Autodesk Inventor part; units mm, degrees
ref_plane "Work Plane1" through (-12.5, 0, 453) normal (1, 0, 0) x (0, 1, 0)
ref_plane "XZ Plane" through (0, 0, 0) normal (0, 1, 0) x (-1, 0, 0)
ref_plane "XY Plane" through (0, 0, 0) normal (0, 0, 1) x (1, 0, 0)
sketch "Sketch2" plane through (0, 0, 0) normal (0, 1, 0) x (-1, 0, 0)
  line L0 (0, 0) -> (0, 513)
  line L1 (0, 513) -> (-12.5, 513)
  line L2 (-12.5, 513) -> (-12.5, 393)
  line L3 (-19, 393) -> (-19, 308)
  line L4 (-19, 308) -> (-15, 308)
  line L5 (-15, 308) -> (-15, 0)
  line L6 (-15, 0) -> (0, 0)
  line L7 (-19, 393) -> (-12.5, 393)
  dimension "d6" = 30
  dimension "d11" = 308
  dimension "d12" = 85
  dimension "d13" = 120
  dimension "d14" = 38
  dimension "d15" = 25
revolve "Revolution1" add sketch "Sketch2" angle 360 about axis through (0, 0, 0) along (0, 0, 1)
ref_plane "Work Plane1" through (-12.5, 0, 453) normal (1, 0, 0) x (0, 1, 0)
sketch "Sketch3" plane through (-12.5, 0, 453) normal (1, 0, 0) x (0, 1, 0)
  line L0 (12.5, -60) -> (-12.5, -60)
  line L1 (12.5, 60) -> (-12.5, 60)
  line L2 (0.1403, 48) -> (0.1403, 38) construction
  line L3 (-3.8597, 48) -> (-3.8597, 38)
  line L4 (4.1403, 38) -> (4.1403, 48)
  arc A0 (4.1403, 48) -> (-3.8597, 48) centre (0.1403, 48) ccw
  arc A1 (-3.8597, 38) -> (4.1403, 38) centre (0.1403, 38) ccw
  point P0 (0, -453)
  point P1 (0.1403, 43)
  dimension "d8" = 12
  dimension "d9" = 8
  dimension "d10" = 10
extrude "Extrusion2" cut sketch "Sketch3" along normal blind 10
properties part number "NVPH-312 augur shaft"
CAD build for the part. Positions are in the model's coordinates, mm. A direction names the side the tool comes from. Round coordinates to 2 decimals unless told otherwise and drop trailing zeros. Write each loop counter-clockwise with the first axis right and the second up, starting at its lowest first coordinate (ties: lowest second). Pieces come first, ordered by that corner, then holes.
Item 1: Mould opens along Z. For faces 1 (the cylindrical face through (8.767, 16.856, 349.905)), 2 (the flat face through (0, 0, 0)), 3 (the flat face through (0, 0, 513)), 4 (the flat face through (-2.5, 0, 496)) say: released by +Z, released by -Z, zero draft, split by the parting line, or undercut.
Filled in:
face 1: zero draft
face 2: released by -Z
face 3: released by +Z
face 4: undercut
Item 2: Band-saw the part on B-B on z = 416.5. Write the cut outline in (x, y), then the cut area to 3 significant figures.
Filled in:
outline: circle Ø25 at (0, 0)
area: 491 mm2
Item 3: Band-saw the part on A-A on z = 212. Write the cut outline in (x, y), then the cut area to 3 significant figures.
Filled in:
outline: circle Ø30 at (0, 0)
area: 707 mm2
Item 4: Tool access for faces 5 (the flat face through (-7, 4.14, 496)), 6 (the flat face through (14, 6, 308)), 7 (the cylindrical face through (11.923, -3.755, 452.16)): list every direction of +Z, -Z, +X, -X, +Y, -Y with a clear straight run to the whole face (end or side of a thin tool).
Filled in:
face 5: -X
face 6: -Z
face 7: +Z
Item 5: Drill centre lines: L1, parallel to Z at x = -5.5, y = -0.5; L2, parallel to Z at x = 15, y = -6; L3, parallel to Z at x = 3, y = 13.5. Where is each one in solid material? Low to high.
Filled in:
L1: z = 0 to 487.05, 504.95 to 513
L2: z = 308 to 393
L3: z = 0 to 393
Item 6: Drop flat-ended pins along their axis: pin 1 Ø2.5 at (y, z) = (1.5, 497) entering from -X; pin 2 Ø1 at (x, z) = (-12, 104) entering from +Y; pin 3 Ø5 at (y, z) = (-11, 457) entering from +X. Give the stop position or say it passes through.
Filled in:
pin 1: stops at x = -2.5
pin 2: stops at y = 9.63
pin 3: stops at x = 9.17
